Part model, mm, in its own coordinate system. Give positions to 0.01 mm unless a question says otherwise; leave off trailing zeros. Loops run counter-clockwise (first coordinate to the right, second up) from the corner with the lowest first, then second, coordinate; pieces in that order, holes last. Notation, with made-up numbers: (-32.5, 8) -> (2.5, 8) arc R19 cw to (2.5, 42) -> close; hole circle Ø10 at (45.25, 88). An arc over 180 degrees is marked (long way). Write item = value, one per line.
from build123d import *

# Parameters (mm, degrees)
SKETCH001_W         = 501.65
SKETCH001_H         = 508
SKETCH001_R         = 3.81
SKETCH001_W_2       = 177.8
SKETCH001_H_2       = 406.4
PAD007_DEPTH        = 6.35
SKETCH005_W         = 158.75
SKETCH005_H         = 38.1
POCKET_DEPTH        = 6.35
LINEARPATTERN_COUNT = 7
LINEARPATTERN_PITCH = 50.8


with BuildPart() as part:
    # Sketch001 → Pad007 (new body)
    with BuildSketch(Plane(origin=(914.4, 1422.4, 914.4), x_dir=(0, 1, 0), z_dir=(-1, 0, 0))):
        Rectangle(SKETCH001_W, SKETCH001_H)
        with Locations((80.16875, 203.2)):
            Circle(SKETCH001_R, mode=Mode.SUBTRACT)
        with Locations((148.43125, 203.2)):
            Circle(SKETCH001_R, mode=Mode.SUBTRACT)
        with Locations((80.16875, -203.2)):
            Circle(SKETCH001_R, mode=Mode.SUBTRACT)
        with Locations((148.43125, -203.2)):
            Circle(SKETCH001_R, mode=Mode.SUBTRACT)
        with Locations((-111.125, 0)):
            Rectangle(SKETCH001_W_2, SKETCH001_H_2, mode=Mode.SUBTRACT)
    extrude(amount=PAD007_DEPTH)

    # Sketch005 → Pocket (cut)
    with BuildSketch(Plane(origin=(914.4, 1422.4, 914.4), x_dir=(0, 1, 0), z_dir=(1, 0, 0))):
        with Locations((98.425, 158.75)):
            Rectangle(SKETCH005_W, SKETCH005_H)
    pocket = extrude(amount=-POCKET_DEPTH, mode=Mode.SUBTRACT)

    # LinearPattern: Pocket ×7
    with Locations(*[(0, 0, -i * LINEARPATTERN_PITCH) for i in range(1, LINEARPATTERN_COUNT)]):
        add(pocket, mode=Mode.SUBTRACT)


solid = part.part
1) Drop a flat-ended pin along its axis: P1, Ø7, axis at y = 1570.83, z = 1117.6, coming from the -X side. Give the stop position or say it passes through.
Resolved:
P1 = through
2) Slice it at C-C, the plane z = 857.5. List the corners of the cut face in (x, y) (3 decimals).
Resolved:
outline = (908.05, 1171.575) -> (914.4, 1171.575) -> (914.4, 1222.375) -> (908.05, 1222.375) -> close; (908.05, 1400.175) -> (914.4, 1400.175) -> (914.4, 1441.45) -> (908.05, 1441.45) -> close; (908.05, 1600.2) -> (914.4, 1600.2) -> (914.4, 1673.225) -> (908.05, 1673.225) -> close
3) Slice it at D-D, the plane z = 733.5. List the corners of the cut face in (x, y) (3 decimals).
Resolved:
outline = (908.05, 1171.575) -> (914.4, 1171.575) -> (914.4, 1222.375) -> (908.05, 1222.375) -> close; (908.05, 1400.175) -> (914.4, 1400.175) -> (914.4, 1673.225) -> (908.05, 1673.225) -> close
4) Slice it at A-A, the plane y = 1317.5. List the corners of the cut face in (x, z).
Resolved:
outline = (908.05, 660.4) -> (914.4, 660.4) -> (914.4, 711.2) -> (908.05, 711.2) -> close; (908.05, 1117.6) -> (914.4, 1117.6) -> (914.4, 1168.4) -> (908.05, 1168.4) -> close
5) Drill centre lines: line 1 along Y through (x, z) = (912, 785) (3 decimals); line 2 along Z through (x, y) = (913.5, 1324); line 3 along Y through (x, z) = (911.5, 735) (3 decimals). Where is each one in solid material? Low to high. Write a range as [from, to].
Resolved:
line_1 = [1171.575, 1222.375], [1400.175, 1441.45], [1600.2, 1673.225]
line_2 = [660.4, 711.2], [1117.6, 1168.4]
line_3 = [1171.575, 1222.375], [1400.175, 1673.225]
6) Slice it at B-B, the plane y = 1486. Count the separate pieces of the cut face and the enclosed holes in it, and give its area (3 significant figures).
Resolved:
separate_pieces = 8
enclosed_holes = 0
area = 1,530 mm²
